The listing builds one solid part. Answer for the finished solid, in the listing's coordinates (mm). A direction names the side the tool comes from. Coordinates: 2 decimals unless noted, no trailing zeros. Write each loop counter-clockwise with the first axis right and the second up, starting at its lowest first coordinate (ties: lowest second). Pieces come first, ordered by that corner, then holes. Notation, with made-up numbers: M 42.25,-7 L 65.25,-7 A29 ccw 65.25,26 Z; hole C -15,-17.75 d2. An arc over 180 degrees is marked long. Answer as CSV lines item,"result". Start each with the question number.
Autodesk Inventor part; units mm, degrees
ref_plane "YZ Plane" through (0, 0, 0) normal (1, 0, 0) x (0, 1, 0)
ref_plane "XZ Plane" through (0, 0, 0) normal (0, 1, 0) x (-1, 0, 0)
ref_plane "XY Plane" through (0, 0, 0) normal (0, 0, 1) x (1, 0, 0)
sketch "Sketch1" plane through (0, 0, 0) normal (0, 1, 0) x (-1, 0, 0)
  line L0 (0, 0) -> (22.65, 0)
  line L1 (22.65, 0) -> (22.65, -100)
  line L2 (22.65, -100) -> (0, -100)
  line L3 (0, -100) -> (0, 0)
  dimension "d0" = 22.65
  dimension "d1" = 100
extrude "Extrusion1" add sketch "Sketch1" along normal blind 5
sketch "Sketch2" plane through (0, 5, 0) normal (0, 1, 0) x (1, 0, 0)
  line L0 (-22.65, 0) -> (0, 0)
  line L1 (0, 0) -> (0, 100)
  line L2 (-22.65, 0) -> (0, 0)
  line L3 (0, 0) -> (0, 5)
  line L4 (0, 5) -> (-22.65, 5)
  line L5 (-22.65, 5) -> (-22.65, 0)
  line L6 (-22.65, 100) -> (-22.65, 0)
  line L7 (-22.65, 100) -> (0, 100)
  line L8 (0, 100) -> (0, 95)
  line L9 (0, 95) -> (-22.65, 95)
  line L10 (-22.65, 95) -> (-22.65, 100)
  dimension "d4" = 5
  dimension "d5" = 5
extrude "Extrusion2" add sketch "Sketch2" along normal blind 40 contours L5 L4 L1 L0 | L6 L7 L1 L9
sketch "Sketch3" plane through (-22.65, 0, 0) normal (0, 0, 1) x (1, 0, 0)
  point P0 (22.65, 0)
sketch "Sketch4" plane through (-22.65, 0, 0) normal (0, 0, 1) x (1, 0, 0)
  line L0 (22.65, 0) -> (0, 0)
  line L1 (22.65, 0) -> (0, 0)
  line L2 (0, 0) -> (11.325, 0)
  line L3 (11.325, 0) -> (11.325, 45)
  line L4 (22.65, 45) -> (0, 45)
  line L5 (0, 5) -> (22.65, 5)
  line L6 (22.65, 5) -> (0, 5)
  line L7 (11.325, 5) -> (11.325, 15) construction
  dimension "d8" = 10
hole "Hole1" at (-11.325, 15, 0) direction (0, 0, -1) diameter 4 depth 115 tip angle 118
sketch "Sketch5" plane through (-22.65, 0, 0) normal (0, 0, 1) x (1, 0, 0)
  line L0 (0, 5) -> (0, 45)
  line L1 (0, 45) -> (23, 45)
  line L2 (23, 45) -> (23, 21.7538)
  line L3 (23, 21.7538) -> (0, 21.7538)
  line L4 (0, 21.7538) -> (0, 45)
  point P0 (22.65, 0)
  dimension "d16" = 23
extrude "Extrusion3" cut sketch "Sketch5" against normal blind 102.75
sketch "Sketch6" plane through (0, 5, 0) normal (0, 1, 0) x (1, 0, 0)
  line L0 (0, 95) -> (-22.65, 95) construction
  line L1 (-22.65, 5) -> (0, 5) construction
  line L2 (0, 95) -> (0, 5) construction
  line L3 (0, 5) -> (-1.175, 5) construction
  line L4 (-1.175, 5) -> (-1.175, 95) construction
  line L5 (-1.175, 50) -> (-22.65, 50) construction
  line L6 (-22.65, 95) -> (-22.65, 5) construction
  line L7 (0, 5) -> (0, 95) construction
  line L8 (0, 5) -> (-22.65, 5) construction
  line L9 (-13.325, 5) -> (-9.325, 5) construction
  line L10 (-11.325, 5) -> (-11.325, 95) construction
  line L11 (-11.325, 50) -> (-2.825, 50) construction
  line L12 (-2.825, 50) -> (-2.825, 71) construction
  line L13 (-11.325, 50) -> (-19.825, 50) construction
  line L14 (-11.325, 50) -> (-2.825, 50) construction
  line L15 (-19.825, 50) -> (-19.825, 29) construction
  point P0 (0, 0)
  dimension "d19" = 1.175
  dimension "d20" = 8.5
  dimension "d21" = 21
  dimension "d22" = 90
  dimension "d23" = 8.5
  dimension "d24" = 180
  dimension "d25" = 21
hole "Hole2" at (-2.825, 5, -71) at (-19.825, 5, -29) direction (0, -1, 0) diameter 4 depth 115 tip angle 118
fillet "Fillet1" radius 1 2 edges at (-2.825, 5, -73) (-19.825, 5, -31)
sketch "Sketch7" plane through (0, 5, 0) normal (0, 1, 0) x (1, 0, 0)
  circle A0 centre (-2.825, 71) radius 2 construction
  line L0 (-2.825, 71) -> (-22.65, 71) construction
  line L1 (-22.65, 0) -> (-22.65, 100) construction
  circle A1 centre (-19.825, 29) radius 2 construction
  line L2 (-19.825, 29) -> (-19.825, 32.5) construction
  line L3 (-19.825, 32.5) -> (-35.65, 32.5) construction
  line L4 (-22.65, 32.5) -> (-32.65, 32.5) construction
  line L5 (-32.65, 32.5) -> (-32.65, 42.5) construction
  line L6 (-32.65, 42.5) -> (-22.65, 42.5) construction
  line L7 (-22.65, 42.5) -> (-22.65, 32.5) construction
  line L8 (-22.65, 42.5) -> (-32.65, 42.5)
  line L9 (-32.65, 42.5) -> (-32.65, 32.5)
  line L10 (-32.65, 32.5) -> (-22.65, 32.5)
  line L11 (-22.65, 32.5) -> (-22.65, 42.5)
  point P0 (0, 0)
  dimension "d34" = 3.5
  dimension "d35" = 15.825
  dimension "d36" = 10
  dimension "d37" = 10
extrude "Extrusion4" add sketch "Sketch7" against normal blind 5
sketch "Sketch8" plane through (0, 5, 0) normal (0, 1, 0) x (1, 0, 0)
  line L0 (-32.65, 42.5) -> (-22.65, 42.5)
  line L1 (-22.65, 32.5) -> (-32.65, 32.5)
  line L2 (-32.65, 42.5) -> (-27.65, 42.5)
  line L3 (-27.65, 42.5) -> (-27.65, 32.5)
  line L4 (-27.65, 32.5) -> (-32.65, 32.5)
  line L5 (-32.65, 32.5) -> (-32.65, 42.5)
  point P0 (0, 0)
  dimension "d40" = 5
extrude "Extrusion5" add sketch "Sketch8" along normal blind 12.5
sketch "Sketch9" plane through (-32.65, 0, -42.5) normal (-1, 0, 0) x (0, 0, 1)
  line L0 (0, 17.5) -> (0, 0) construction
  line L1 (0, 17.5) -> (5, 17.5) construction
  line L2 (10, 17.5) -> (0, 17.5) construction
  line L3 (10, 0) -> (0, 0) construction
  line L4 (5, 0) -> (5, 17.5) construction
  point P0 (42.5, 0)
  point P1 (5, 12.5)
hole "Hole3" at (-32.65, 12.5, -37.5) direction (1, 0, 0) diameter 6 depth 115 tip angle 118
fillet "Fillet2" radius 7 4 edges at (-22.65, 21.7538, -97.5) (-22.65, 21.7538, -2.5) (0, 21.7538, -2.5) (0, 21.7538, -97.5)
properties part number "mtv_axelHolder(pushingAxel)1-13"
1) The part is cut by section D-D (z = -16.5). Determine the outline of the cut face in (x, y), then the cut area to 3 significant figures.
2) Each of these flat-tipped pins is pushed along its axis until it touches: P1, Ø12, axis at y = 4.5, z = -23.5, coming from the -X side; P2, Ø1.5, axis at x = -9.5, z = -60.5, coming from the +Y side; P3, Ø1.5, axis at x = -31.5, z = -39.5, coming from the +Y side. Where does it stop, or does it pass through?
3) The part is cut by section B-B (x = -8). Determine the outline of the cut face in (y, z).
4) The part is cut by section A-A (y = 8.5). Determine the outline of the cut face in (x, z), then the cut area to 4 significant figures.
5) For a pull along X with two mould halves and no side action, classify faces 4 (the face through (-2, 19.65, -97.46)), 5 (the face through (-10.11, 16.59, -97.54)), 6 (the face through (-30.1, 12.4, -40.5)), 7 (the face through (-3.426, 1.98, -69.092)) as +X half, -X half, draft (parallel to the pull), parting line (faces both ways), or undercut.
6) The part is cut by section C-C (z = -37.5). Determine the outline of the cut face in (x, y), then the cut area to 3 significant figures.
7) Find the intervals of material crossed by line 1 (X direction, y = 3.15, z = -71) (3 decimals); line 2 (X direction, y = 15, z = -98.25) (3 decimals); line 3 (Z direction, x = -19, y = 7.25), in increasing order. Write a range as from..to.
8) Which of the six approach directions +Z, -Z, +X, -X, +Y, -Y give full straight-line access (tool end or side, diameter ignored) to faces 1 (the face through (-29, 7, -42.5)), 2 (the face through (-11, 11, -5)), 3 (the face through (-27.65, 8, -38))?
Completed:
1,outline,"M -22.65,0 L 0,0 L 0,5 L -22.65,5 Z"
1,area,"113 mm²"
2,P1,"x = -22.65"
2,P2,"y = 5"
2,P3,"y = 17.5"
3,outline,"M 0,-100 L 21.75,-100 L 21.75,-95 L 5,-95 L 5,-5 L 21.75,-5 L 21.75,0 L 0,0 Z"
4,outline,"M -32.65,-42.5 L -27.65,-42.5 L -27.65,-32.5 L -32.65,-32.5 Z; M -22.65,-100 L 0,-100 L 0,-95 L -22.65,-95 Z; M -22.65,-5 L 0,-5 L 0,0 L -22.65,0 Z"
4,area,"276.5 mm²"
5,face 4,"+X half"
5,face 5,"undercut"
5,face 6,"draft"
5,face 7,"undercut"
6,outline,"M -32.65,0 L 0,0 L 0,5 L -27.65,5 L -27.65,9.5 L -32.65,9.5 Z; M -32.65,15.5 L -27.65,15.5 L -27.65,17.5 L -32.65,17.5 Z"
6,area,"196 mm²"
7,line 1,"-22.65..-4.825, -0.825..0"
7,line 2,"-22.646..-13.325, -9.325..-0.004"
7,line 3,"-100..-95, -5..0"
8,face 1,"-Z, -X, +Y, -Y"
8,face 2,"+X, -X, +Y"
8,face 3,"+Z, -Z, +X, +Y"
